```python
from build123d import *

# Parameters (mm, degrees)
SKETCH1_W           = 150
SKETCH1_H           = 150
BOSS_EXTRUDE1_DEPTH = 2.5
CUT_EXTRUDE1_DEPTH  = 5
SKETCH3_R           = 1.55
CUT_EXTRUDE2_DEPTH  = 5
SKETCH4_R           = 5.25
SKETCH4_W           = 30
SKETCH4_H           = 18
CUT_EXTRUDE3_DEPTH  = 5
FILLET1_R           = 1


with BuildPart() as part:
    # Sketch1 → Boss-Extrude1 (new body, symmetric)
    with BuildSketch(Plane(origin=(0, 0, 0), x_dir=(1, 0, 0), z_dir=(0, 1, 0))):
        Rectangle(SKETCH1_W, SKETCH1_H)
    extrude(amount=BOSS_EXTRUDE1_DEPTH, both=True)

    # Sketch2 → Cut-Extrude1 (cut)
    with BuildSketch(Plane(origin=(0, 2.5, 0), x_dir=(1, 0, 0), z_dir=(0, 1, 0))):
        Polygon((50.251262658, 75), (75, 75), (75, 50.251262658), align=None)
        Polygon((-75, 75), (-75, 50.251262658), (-50.251262658, 75), align=None)
        Polygon((-50.251262658, -75), (-75, -75), (-75, -50.251262658), align=None)
        Polygon((75, -75), (75, -50.251262658), (50.251262658, -75), align=None)
    extrude(amount=-CUT_EXTRUDE1_DEPTH, mode=Mode.SUBTRACT)

    # Sketch3 → Cut-Extrude2 (cut)
    with BuildSketch(Plane(origin=(0, 2.5, 0), x_dir=(1, 0, 0), z_dir=(0, 1, 0))):
        with Locations((69.343145751, 50.251262658)):
            Circle(SKETCH3_R)
        with Locations((53.786796564, 34.694913472)):
            Circle(SKETCH3_R)
        with Locations((34.694913472, 53.786796564)):
            Circle(SKETCH3_R)
        with Locations((50.251262658, 69.343145751)):
            Circle(SKETCH3_R)
        with Locations((-69.343145751, 50.251262658)):
            Circle(SKETCH3_R)
        with Locations((-53.786796564, 34.694913472)):
            Circle(SKETCH3_R)
        with Locations((-34.694913472, 53.786796564)):
            Circle(SKETCH3_R)
        with Locations((-50.251262658, 69.343145751)):
            Circle(SKETCH3_R)
        with Locations((-53.786796564, -34.694913472)):
            Circle(SKETCH3_R)
        with Locations((-69.343145751, -50.251262658)):
            Circle(SKETCH3_R)
        with Locations((-34.694913472, -53.786796564)):
            Circle(SKETCH3_R)
        with Locations((-50.251262658, -69.343145751)):
            Circle(SKETCH3_R)
        with Locations((69.343145751, -50.251262658)):
            Circle(SKETCH3_R)
        with Locations((53.786796564, -34.694913472)):
            Circle(SKETCH3_R)
        with Locations((34.694913472, -53.786796564)):
            Circle(SKETCH3_R)
        with Locations((50.251262658, -69.343145751)):
            Circle(SKETCH3_R)
    extrude(amount=-CUT_EXTRUDE2_DEPTH, mode=Mode.SUBTRACT)

    # Sketch4 → Cut-Extrude3 (cut)
    with BuildSketch(Plane(origin=(0, 2.5, 0), x_dir=(1, 0, 0), z_dir=(0, 1, 0))):
        with Locations((17, -17)):
            Circle(SKETCH4_R)
        with Locations((17, 17)):
            Circle(SKETCH4_R)
        with Locations((-17, -17)):
            Circle(SKETCH4_R)
        with Locations((-17, 17)):
            Circle(SKETCH4_R)
        Rectangle(SKETCH4_W, SKETCH4_H)
    extrude(amount=-CUT_EXTRUDE3_DEPTH, mode=Mode.SUBTRACT)

    # Fillet1
    fillet1_edges = [part.edges().sort_by_distance(p)[0] for p in [
        (-15, 0, 9),
        (-15, 0, -9),
        (15, 0, -9),
        (15, 0, 9),
    ]]
    fillet(fillet1_edges, radius=FILLET1_R)


solid = part.part
```
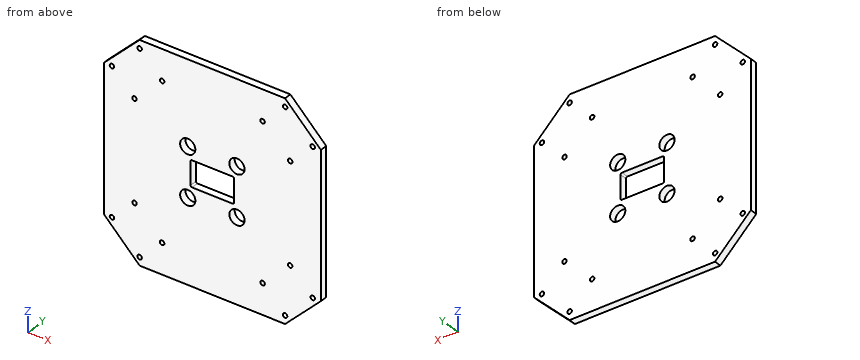
The listing builds one solid part. Answer for the finished solid, in the listing's coordinates (mm). Round coordinates to 2 decimals unless told otherwise and drop trailing zeros. Write each loop counter-clockwise with the first axis right and the second up, starting at its lowest first coordinate (ties: lowest second). Pieces come first, ordered by that corner, then holes. Notation, with made-up numbers: (-22, -30.75) -> (28, -30.75) arc R26 cw to (28, -4.75) -> close; hole circle Ø8 at (-11, 15). An arc over 180 degrees is marked (long way). Answer as a JSON object with one key per item and string values. Group by question number.
Q1. Straight lines are drawn through the part: line 1 along Z through (x, y) = (-4.5, 0.6); line 2 along Z through (x, y) = (17, 1.2); line 3 along X through (y, z) = (0.2, 52.5). For each, find the intervals that lie inside material, in ascending order.
Q2. Section D-D (x = 63) is taken. Write down the section's boundary in (y, z).
Q3. Section B-B (x = -3.5) is taken. Write down the section's boundary in (y, z).
Q4. Section C-C (y = -0.5) is taken. Count the separate pieces of the cut face and the enclosed holes in it, plus the area to 3 significant figures.
Q5. Section A-A (z = -17) is taken. Write down the section's boundary in (x, y).
Check values:
{
 "1": {"line 1": "-75 to -9, 9 to 75", "line 2": "-75 to -22.25, -11.75 to 11.75, 22.25 to 75", "line 3": "-72.75 to -35.56, -33.83 to 33.83, 35.56 to 72.75"},
 "2": {"outline": "(-2.5, -62.25) -> (2.5, -62.25) -> (2.5, 62.25) -> (-2.5, 62.25) -> close"},
 "3": {"outline": "(-2.5, -75) -> (2.5, -75) -> (2.5, -9) -> (-2.5, -9) -> close; (-2.5, 9) -> (2.5, 9) -> (2.5, 75) -> (-2.5, 75) -> close"},
 "4": {"separate pieces": "1", "enclosed holes": "21", "area": "20,300 mm^2"},
 "5": {"outline": "(-75, -2.5) -> (-22.25, -2.5) -> (-22.25, 2.5) -> (-75, 2.5) -> close; (-11.75, -2.5) -> (11.75, -2.5) -> (11.75, 2.5) -> (-11.75, 2.5) -> close; (22.25, -2.5) -> (75, -2.5) -> (75, 2.5) -> (22.25, 2.5) -> close"}
}
